CAD build for the part. Positions are in the model's coordinates, mm. Give positions to 0.01 mm unless a question says otherwise; leave off trailing zeros. Write each loop counter-clockwise with the first axis right and the second up, starting at its lowest first coordinate (ties: lowest second). Pieces come first, ordered by that corner, then holes. Notation, with made-up numbers: (12, 8.5) - (48, 8.5) arc R31 ccw to (48, 46.5) - close; hole circle Ø8 at (12, -22). An arc over 180 degrees is marked (long way). Answer as a JSON object with one key per item and string values.
from build123d import *

# Parameters (mm, degrees)
F0_R     = 3
F0_R_2   = 2
F1_DEPTH = 5
F2_R     = 1
F3_SIZE  = 1


with BuildPart() as f1:
    # F0 (on Right) → F1 (new body)
    with BuildSketch(Plane.YZ):
        with BuildLine():
            ThreePointArc((57.72593, -60.441806), (60.927082, -55.222327), (59.49991, -49.268042))
            Line((59.49991, -49.268042), (-13.845659, 51.761887))
            ThreePointArc((-13.845659, 51.761887), (-18.475487, 56.562027), (-24.247485, 59.902791))
            Line((-24.247485, 59.902791), (-56.768679, 73.091937))
            ThreePointArc((-56.768679, 73.091937), (-64.583772, 69.786739), (-61.278574, 61.971647))
            Line((-61.278574, 61.971647), (-28.757379, 48.7825))
            ThreePointArc((-28.757379, 48.7825), (-25.87138, 47.112118), (-23.556466, 44.712049))
            Line((-23.556466, 44.712049), (26.902381, -24.792543))
            ThreePointArc((26.902381, -24.792543), (28.464555, -26.725344), (30.218225, -28.486239))
            ThreePointArc((30.218225, -28.486239), (31.154485, -36.797105), (23.024955, -38.761238))
            ThreePointArc((23.024955, -38.761238), (14.604776, -41.953407), (18.827654, -49.906813))
            ThreePointArc((18.827654, -49.906813), (20.17817, -50.271255), (21.505159, -50.713759))
            Line((21.505159, -50.713759), (51.487555, -61.692687))
            ThreePointArc((51.487555, -61.692687), (54.378812, -62.001114), (57.075581, -60.913946))
            Line((57.075581, -60.913946), (57.72593, -60.441806))
        make_face()
        with Locations((20.221904, -44.068756)):
            Circle(F0_R, mode=Mode.SUBTRACT)
        with Locations((53.026038, -53.967934)):
            Circle(F0_R, mode=Mode.SUBTRACT)
        with Locations((-59.023626, 67.531792)):
            Circle(F0_R_2, mode=Mode.SUBTRACT)
    extrude(amount=F1_DEPTH)

    # F2
    f2_edges = [f1.edges().sort_by_distance(p)[0] for p in [
        (0, -40.508082, 66.497364),
        (5, -40.508082, 66.497364),
    ]]
    fillet(f2_edges, radius=F2_R)

    # F3
    f3_edges = [f1.edges().sort_by_distance(p)[0] for p in [
        (5, 17.221904, -44.068756),
        (0, 17.221904, -44.068756),
        (5, 50.026038, -53.967934),
        (0, 50.026038, -53.967934),
        (0, -61.023626, 67.531792),
        (5, -61.023626, 67.531792),
    ]]
    chamfer(f3_edges, length=F3_SIZE)


solid = f1.part
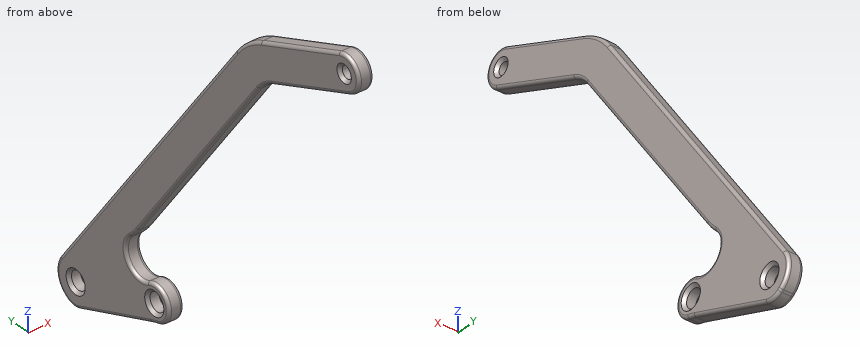
(1) Flat gauge pins, fed straight in: P1, Ø6, axis at y = -7, z = 14.5, coming from the -X side (3 decimals); P2, Ø1, axis at x = 1, z = 31, coming from the -Y side; P3, Ø4.5, axis at y = -59.02, z = 67.53, coming from the +X side; P4, Ø1, axis at x = 4, z = 22, coming from the +Y side. Where does each tip first touch, or does it go through?
Answer key:
{"P1": "passes through", "P2": "stops at y = -13.96", "P3": "stops at x = 4.25", "P4": "stops at y = 8.12"}
(2) Saw through at A-A, the plane x = 2.4. Give the cut face in (y, z).
Answer key:
{"outline": "(-61.28, 61.97) - (-28.76, 48.78) arc R12 cw to (-23.56, 44.71) - (26.9, -24.79) arc R24 ccw to (30.22, -28.49) arc R6.32 cw to (23.02, -38.76) arc R6 ccw (long way) to (18.83, -49.91) arc R24 cw to (21.51, -50.71) - (51.49, -61.69) arc R6 ccw to (57.08, -60.91) - (57.73, -60.44) arc R8 ccw to (59.5, -49.27) - (-13.85, 51.76) arc R24 ccw to (-24.25, 59.9) - (-56.77, 73.09) arc R6 ccw to start; hole circle Ø4 at (-59.02, 67.53); hole circle Ø6 at (20.22, -44.07); hole circle Ø6 at (53.03, -53.97)"}
(3) Probe L1, parallel to Y at x = 4.35, z = -39; L2, parallel to Y at x = 4.5, z = -41; L3, parallel to Z at x = 3.15, y = 25. List the from-to ranges inside material, lowest first. Write a range as [from, to].
Answer key:
{"L1": "y = [17.13, 23.37], [28.58, 51.97]", "L2": "y = [15.22, 18.54], [21.9, 53.33]", "L3": "z = [-51.99, -39.42], [-22.17, -1.75]"}
